from build123d import *

# Parameters (mm, degrees)
SKETCH1_R           = 4.88
BOSS_EXTRUDE1_DEPTH = 0.2
BOSS_EXTRUDE2_DEPTH = 0.001


with BuildPart() as part:
    # Sketch1 → Boss-Extrude1 (new body)
    with BuildSketch(Plane.XY):
        with Locations((-24.02000111, -6.774872108)):
            Circle(SKETCH1_R)
    extrude(amount=BOSS_EXTRUDE1_DEPTH)

    # Sketch3 → Boss-Extrude2 (add)
    with BuildSketch(Plane.XY.offset(0.2)):
        with BuildLine():
            Line((-24.836675582, -8.155782129), (-24.836675582, -4.655782129))
            Line((-24.836675582, -4.655782129), (-24.275778146, -4.655782129))
            add(Edge.make_bspline(
                [(-24.275778146, -4.655782129), (-24.236511819, -4.655777648), (-24.160532219, -4.655768977), (-24.050913486, -4.659618427), (-23.949251368, -4.664598122), (-23.855869395, -4.670169242), (-23.770608623, -4.679769396), (-23.693598705, -4.68988691), (-23.624685775, -4.702088007), (-23.582080655, -4.71303277), (-23.562036159, -4.718181969)],
                knots=[0, 0, 0, 0, 1.311965854, 2.538629056, 3.664479157, 4.713267157, 5.663616078, 6.530575999, 7.308677837, 8, 8, 8, 8], degree=3))
            add(Edge.make_bspline(
                [(-23.562036159, -4.718181969), (-23.535715701, -4.725445006), (-23.484066512, -4.739697417), (-23.410088391, -4.768480776), (-23.339909823, -4.800475521), (-23.273616496, -4.836975541), (-23.211615476, -4.878421493), (-23.154142389, -4.925142306), (-23.099957682, -4.975262607), (-23.05098533, -5.030179235), (-23.006722392, -5.088208826), (-22.968265836, -5.149336173), (-22.934852017, -5.2126266), (-22.90811221, -5.278876575), (-22.887964268, -5.347780999), (-22.873228147, -5.419045639), (-22.863677145, -5.492895994), (-22.8627747, -5.543138805), (-22.862316608, -5.568642706)],
                knots=[0, 0, 0, 0, 1.099996261, 2.158545794, 3.195537121, 4.207578794, 5.205712374, 6.197378256, 7.190519799, 8.17788031, 9.159561366, 10.129234751, 11.085776129, 12.040971148, 13.00380137, 13.975669004, 14.972423361, 16, 16, 16, 16], degree=3))
            add(Edge.make_bspline(
                [(-22.862316608, -5.568642706), (-22.863514384, -5.601408525), (-22.865872058, -5.665904014), (-22.880933042, -5.760636218), (-22.909174734, -5.850171768), (-22.946128301, -5.936160769), (-22.996373599, -6.018282481), (-23.06017541, -6.096497859), (-23.136500353, -6.17321527), (-23.195045798, -6.219202183), (-23.225497698, -6.243121873)],
                knots=[0, 0, 0, 0, 0.986156485, 1.941127874, 2.875419072, 3.804401753, 4.751181392, 5.761612777, 6.835722519, 8, 8, 8, 8], degree=3))
            add(Edge.make_bspline(
                [(-23.225497698, -6.243121873), (-23.200820939, -6.255719144), (-23.152436643, -6.280418908), (-23.083745156, -6.321017946), (-23.020144338, -6.364200172), (-22.961349022, -6.409096743), (-22.908592505, -6.457610888), (-22.859696385, -6.506947156), (-22.81707294, -6.559932311), (-22.778957771, -6.61467786), (-22.745828686, -6.671976526), (-22.716976906, -6.731731543), (-22.692606843, -6.794147048), (-22.671969642, -6.858905396), (-22.656578413, -6.926229327), (-22.646543004, -6.996142917), (-22.638859268, -7.068407727), (-22.638261545, -7.11763271), (-22.637957634, -7.142661136)],
                knots=[0, 0, 0, 0, 1.164658916, 2.283573913, 3.35186032, 4.395461096, 5.390182219, 6.362969632, 7.312859996, 8.245001507, 9.165155236, 10.092416118, 11.032087915, 11.979892451, 12.947605196, 13.931445124, 14.948243989, 16, 16, 16, 16], degree=3))
            add(Edge.make_bspline(
                [(-22.637957634, -7.142661136), (-22.639929818, -7.190463998), (-22.643821916, -7.284802755), (-22.672279037, -7.423313716), (-22.721614642, -7.554634671), (-22.787862186, -7.678243692), (-22.869491907, -7.790562503), (-22.963342678, -7.888952806), (-23.068469636, -7.972238013), (-23.16546196, -8.028449067), (-23.249352683, -8.06617194), (-23.318837801, -8.0894946), (-23.393463346, -8.111100676), (-23.474596277, -8.126272909), (-23.560765765, -8.140160205), (-23.652811968, -8.148734509), (-23.750562854, -8.154545104), (-23.817702388, -8.155361451), (-23.852300582, -8.155782129)],
                knots=[0, 0, 0, 0, 1.284142165, 2.534249414, 3.780121997, 5.041676246, 6.291546858, 7.49970053, 8.684500223, 9.883330709, 10.50184324, 11.153274765, 11.851151195, 12.587658647, 13.369265475, 14.195992086, 15.070362669, 16, 16, 16, 16], degree=3))
            Line((-23.852300582, -8.155782129), (-24.836675582, -8.155782129))
        make_face()
        with BuildLine():
            Line((-24.208470454, -5.283987258), (-24.208470454, -6.04680777))
            Line((-24.208470454, -6.04680777), (-24.041603467, -6.04680777))
            add(Edge.make_bspline(
                [(-24.041603467, -6.04680777), (-24.018924744, -6.046610003), (-23.975144842, -6.046228226), (-23.911909418, -6.041311067), (-23.853110685, -6.032922088), (-23.798971656, -6.021217352), (-23.748988004, -6.006354044), (-23.70347904, -5.988470283), (-23.662644859, -5.966650151), (-23.615204985, -5.934148102), (-23.565057617, -5.886319881), (-23.520913454, -5.817222107), (-23.494912836, -5.737759929), (-23.492017068, -5.681717049), (-23.490521736, -5.652777322)],
                knots=[0, 0, 0, 0, 1.065314748, 2.056525647, 2.977365736, 3.853934255, 4.656397591, 5.425096493, 6.14721249, 6.826394842, 8.123232004, 9.372140726, 10.643011755, 12, 12, 12, 12], degree=3))
            add(Edge.make_bspline(
                [(-23.490521736, -5.652777322), (-23.491718276, -5.625670459), (-23.494031737, -5.573260429), (-23.520211016, -5.49967208), (-23.560872612, -5.434457742), (-23.608879341, -5.389823861), (-23.654087005, -5.359340236), (-23.692796581, -5.339268067), (-23.735283248, -5.321299666), (-23.782369501, -5.307560589), (-23.833786453, -5.29725127), (-23.889284342, -5.289680309), (-23.948958922, -5.284527191), (-23.990176282, -5.284171096), (-24.01145523, -5.283987258)],
                knots=[0, 0, 0, 0, 1.347982417, 2.606269829, 3.849316587, 5.153353503, 5.842674298, 6.568177932, 7.326619318, 8.142485038, 9.012069166, 9.942760135, 10.937925643, 12, 12, 12, 12], degree=3))
            Line((-24.01145523, -5.283987258), (-24.208470454, -5.283987258))
        make_face(mode=Mode.SUBTRACT)
        with BuildLine():
            Line((-24.208470454, -6.630141104), (-24.208470454, -7.527577001))
            Line((-24.208470454, -7.527577001), (-24.027581031, -7.527577001))
            add(Edge.make_bspline(
                [(-24.027581031, -7.527577001), (-23.991818962, -7.527372694), (-23.923061921, -7.526979887), (-23.824567582, -7.522233852), (-23.735011604, -7.513679959), (-23.654631277, -7.503001112), (-23.583303484, -7.488532946), (-23.521269328, -7.470138526), (-23.467678092, -7.449901461), (-23.422851113, -7.424906282), (-23.386230038, -7.395818093), (-23.353183358, -7.366089264), (-23.326239154, -7.331794252), (-23.304920397, -7.294405246), (-23.286469051, -7.254851016), (-23.275340502, -7.211586983), (-23.266867615, -7.165895389), (-23.266401329, -7.134291502), (-23.266162762, -7.118121873)],
                knots=[0, 0, 0, 0, 1.753078804, 3.370512758, 4.83203934, 6.162291463, 7.344201807, 8.395507345, 9.331626367, 10.147333109, 10.898971645, 11.62040215, 12.321813352, 13.025280112, 13.727906689, 14.453419512, 15.208716525, 16, 16, 16, 16], degree=3))
            add(Edge.make_bspline(
                [(-23.266162762, -7.118121873), (-23.266688872, -7.099631647), (-23.267713593, -7.063617662), (-23.276082503, -7.010979379), (-23.291291546, -6.961838049), (-23.310448079, -6.914937062), (-23.337105411, -6.871955637), (-23.368786739, -6.83140635), (-23.407065872, -6.794662324), (-23.450112989, -6.759501145), (-23.50032319, -6.728715627), (-23.557720031, -6.702003737), (-23.622615324, -6.679694951), (-23.695210087, -6.66193268), (-23.775186072, -6.646858087), (-23.863127016, -6.63785689), (-23.958300515, -6.631162305), (-24.024295368, -6.630489239), (-24.05843039, -6.630141104)],
                knots=[0, 0, 0, 0, 0.845221588, 1.646264278, 2.427170338, 3.19324141, 3.95557735, 4.731569926, 5.540061037, 6.376114724, 7.268642756, 8.224665384, 9.265483498, 10.400594375, 11.639216012, 12.983232105, 14.439614077, 16, 16, 16, 16], degree=3))
            Line((-24.05843039, -6.630141104), (-24.208470454, -6.630141104))
        make_face(mode=Mode.SUBTRACT)
    extrude(amount=BOSS_EXTRUDE2_DEPTH)


solid = part.part
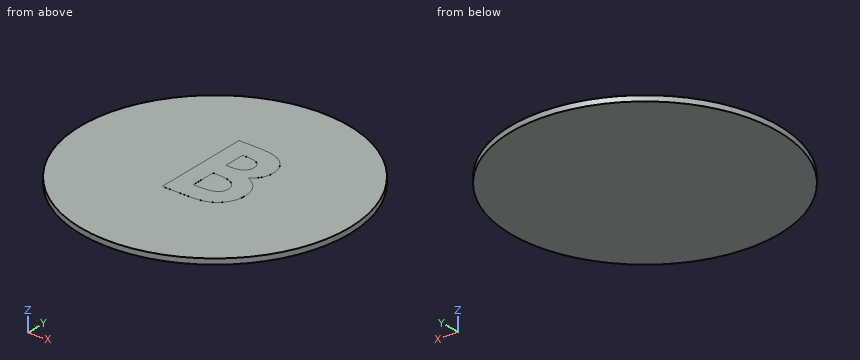
Can you work these out from the model? Positions are in its coordinate system, mm. Coordinates: 2 decimals unless noted, no trailing zeros. Order: outer loops, then holes, each group sorted by start corner. A loop starts at its lowest first (then second) coordinate and runs counter-clockwise, first axis right, second up. Notation, with made-up numbers: (34.5, 4.25) -> (57.5, 4.25) arc R25 cw to (57.5, 43.25) -> close; hole circle Ø8 at (-6, 61). An arc over 180 degrees is marked (long way). Use one line per item in the form item = value.
Q1. Imagine slicing it at A-A, the plane x = -25.75. List the corners of the cut face in (y, z) for me.
From the geometry:
outline = (-11.34, 0) -> (-2.21, 0) -> (-2.21, 0.2) -> (-11.34, 0.2) -> close
Q2. I need wall thicknesses on L1, parallel to Z at x = -26.5, y = -10; L2, parallel to Y at x = -26.5, z = 0.05; L3, parallel to X at y = -6.5, z = 0.1. Which ranges of each line are inside material? Lowest first, please.
From the geometry:
L1 = 0 to 0.2
L2 = -10.98 to -2.57
L3 = -28.89 to -19.15
Q3. Imagine slicing it at C-C, the plane y = -10.75. List the corners of the cut face in (x, z) for me, then the cut area to 3 significant figures.
From the geometry:
outline = (-26.85, 0) -> (-21.19, 0) -> (-21.19, 0.2) -> (-26.85, 0.2) -> close
area = 1.13 mm²
Q4. Imagine slicing it at B-B, the plane z = 0.15. List the corners of the cut face in (x, y) for me.
From the geometry:
outline = circle Ø9.76 at (-24.02, -6.77)
